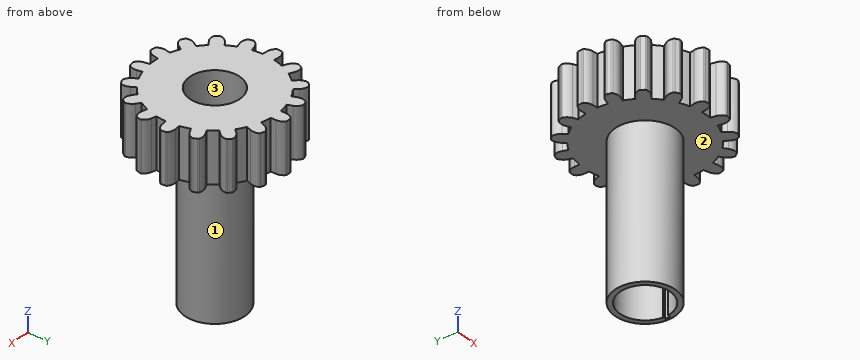
from build123d import *

# Parameters (mm, degrees)
SKETCH1_R           = 24.25521333
BOSS_EXTRUDE1_DEPTH = 10
BOSS_EXTRUDE2_DEPTH = 20
CIRPATTERN1_COUNT   = 17
SKETCH3_R           = 12
CUT_EXTRUDE1_DEPTH  = 20
SKETCH4_R           = 12
SKETCH4_R_2         = 10
BOSS_EXTRUDE3_DEPTH = 80
CUT_EXTRUDE2_START  = -20
CUT_EXTRUDE2_DEPTH  = 20


with BuildPart() as part:
    # Sketch1 → Boss-Extrude1 (new, symmetric)
    with BuildSketch(Plane.XY):
        Circle(SKETCH1_R)
    extrude(amount=BOSS_EXTRUDE1_DEPTH, both=True)

    # Sketch2 → Boss-Extrude2 (add, through all)
    with BuildSketch(Plane.XY.offset(10)):
        with BuildLine():
            Line((2.5, 24.126031039), (2.5, 26.126031039))
            ThreePointArc((2.5, 26.126031039), (2.171151383, 27.721007214), (1.233789603, 29.052714129))
            ThreePointArc((1.233789603, 29.052714129), (0.99677215, 29.202753866), (0.721205098, 29.25521333))
            Line((0.721205098, 29.25521333), (-0.721205098, 29.25521333))
            ThreePointArc((-0.721205098, 29.25521333), (-0.99677215, 29.202753866), (-1.233789603, 29.052714129))
            ThreePointArc((-1.233789603, 29.052714129), (-2.171151383, 27.721007214), (-2.5, 26.126031039))
            Line((-2.5, 26.126031039), (-2.5, 24.126031039))
            ThreePointArc((-2.5, 24.126031039), (0, 24.25521333), (2.5, 24.126031039))
        make_face()
    boss_extrude2 = extrude(amount=-BOSS_EXTRUDE2_DEPTH)

    # CirPattern1: Boss-Extrude2 ×17 about axis
    cirpattern1_axis = Axis((0, 0, 0), (0, 0, 1))
    for i in range(1, CIRPATTERN1_COUNT):
        add(boss_extrude2.rotate(cirpattern1_axis, i * 360 / CIRPATTERN1_COUNT))

    # Sketch3 → Cut-Extrude1 (cut)
    with BuildSketch(Plane.XY.offset(10)):
        Circle(SKETCH3_R)
    extrude(amount=-CUT_EXTRUDE1_DEPTH, mode=Mode.SUBTRACT)

    # Sketch4 → Boss-Extrude3 (add)
    with BuildSketch(Plane.XY.offset(10)):
        Circle(SKETCH4_R)
        Circle(SKETCH4_R_2, mode=Mode.SUBTRACT)
    extrude(amount=-BOSS_EXTRUDE3_DEPTH)

    # Sketch5 → Cut-Extrude2 (cut)
    with BuildSketch(Plane(origin=(0, 0, -70), x_dir=(-1, 0, 0), z_dir=(0, 0, -1)).offset(CUT_EXTRUDE2_START)):
        with BuildLine():
            Line((-10.971006085, 0.760945232), (-10.971006085, -1.239054768))
            Line((-10.971006085, -1.239054768), (-9.922940254, -1.239054768))
            ThreePointArc((-9.922940254, -1.239054768), (-9.997113345, -0.240259783), (-9.971006085, 0.760945232))
            Line((-9.971006085, 0.760945232), (-10.971006085, 0.760945232))
        make_face()
    extrude(amount=CUT_EXTRUDE2_DEPTH, mode=Mode.SUBTRACT)


solid = part.part
Input: part model. Units: mm. Frame: model coordinates. Face numbers are marked on the shaded views. Round coordinates to 2 decimals unless told otherwise and drop trailing zeros. Write each loop counter-clockwise with the first axis right and the second up, starting at its lowest first coordinate (ties: lowest second). Pieces come first, ordered by that corner, then holes.
1) Cut plane C-C (y = -11). Return the cut outline in (x, z), then the cut area to 3 significant figures.
2) Cut plane B-B (z = -36). Return the cut outline in (x, y), then the cut area to 3 significant figures.
3) Draft query along X for the marked faces 1, 2 and 3. Return one class per face: pulls with the +X half, pulls with the -X half, needs draft (parallel to the pull), parting line crosses it, or undercut.
4) Ray query, L1, parallel to Y at x = 0, z = -30; L2, parallel to Z at x = 25, y = 3.5; L3, parallel to Y at x = 5.5, z = -9. Return the intervals inside material, ascending.
5) Cut plane A-A (y = 7). Return the cut outline in (x, z), then the cut area to 3 significant figures.
6) Contact query for flat-ended pins moving along their axis: P1, Ø0.5, axis at x = 10.5, y = 0, coming from the -Z side; P2, Ø0.6, axis at y = 25, z = -4, coming from the -X side; P3, Ø3, axis at y = 5, z = -23, coming from the +X side. Output: stop coordinate, or through.
Geometry says:
1. outline: (-21.62, -10) - (-4.8, -10) - (-4.8, -70) - (4.8, -70) - (4.8, -10) - (21.62, -10) - (21.62, 10) - (-21.62, 10) - close
1. area: 1,440 mm2
2. outline: circle Ø24 at (0, 0); hole circle Ø20 at (0, 0)
2. area: 138 mm2
3. face 1: parting line crosses it
3. face 2: needs draft
3. face 3: undercut
4. L1: y = -12 to -10, 10 to 12
4. L2: z = -10 to 10
4. L3: y = -28.73 to -8.35, 8.35 to 23.62
5. outline: (-23.22, -10) - (-9.75, -10) - (-9.75, -70) - (-7.14, -70) - (-7.14, 10) - (-23.22, 10) - close; (7.14, -70) - (9.75, -70) - (9.75, -10) - (23.22, -10) - (23.22, 10) - (7.14, 10) - close
5. area: 956 mm2
6. P1: stops at z = -50
6. P2: stops at x = -12.04
6. P3: stops at x = 11.48
